Verification items for the finished model (mm, model axes). Coordinates: 2 decimals unless noted, no trailing zeros. Answer in a Markdown table with one row per item.
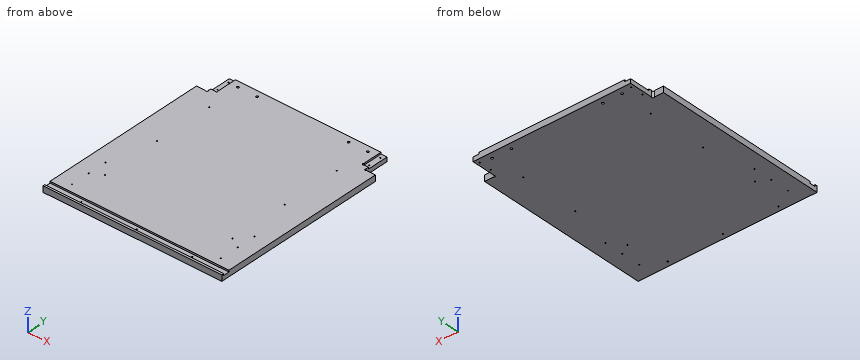
```python
from build123d import *

# Parameters (mm, degrees)
EXTRUDE1_DEPTH     = 17.78
SKETCH4_R          = 3.175
SKETCH4_R_2        = 3.175000003
CUT_EXTRUDE1_DEPTH = 17.78
SKETCH6_R          = 1.5875
CUT_EXTRUDE3_DEPTH = 17.78
SKETCH5_W          = 17.78
SKETCH5_H          = 63.50740041
SKETCH5_H_2        = 63.507400408
CUT_EXTRUDE2_DEPTH = 5.08
SKETCH7_R          = 3.302
CUT_EXTRUDE4_DEPTH = 5.08
SKETCH9_R          = 3.175
CUT_EXTRUDE5_DEPTH = 17.78


with BuildPart() as part:
    # Sketch3 → Extrude1 (new body)
    with BuildSketch(Plane.XY):
        Polygon((10806.641666666, -6342.0625), (11340.041666666, -6342.0625), (11340.041666666, -5818.73683858), (11312.781794728, -5818.73683858), (11308.291666667, -5814.246710519), (11308.291666667, -5742.536838581), (10838.391666667, -5742.536838581), (10838.391666667, -5814.246710519), (10833.901538605, -5818.736838581), (10806.641666666, -5818.736838581), align=None)
    extrude(amount=-EXTRUDE1_DEPTH)

    # Sketch4 → Cut-Extrude1 (cut)
    with BuildSketch(Plane.XY):
        with Locations((11310.536730697, -5816.49177455)):
            Circle(SKETCH4_R)
        with Locations((10836.146602636, -5816.49177455)):
            Circle(SKETCH4_R_2)
    extrude(amount=-CUT_EXTRUDE1_DEPTH, mode=Mode.SUBTRACT)

    # Sketch6 → Cut-Extrude3 (cut)
    with BuildSketch(Plane.XY):
        with Locations((10851.409166666, -6294.4375)):
            Circle(SKETCH6_R)
        with Locations((10908.241666666, -6326.8225)):
            Circle(SKETCH6_R)
        with Locations((11073.341666666, -6326.8225)):
            Circle(SKETCH6_R)
        with Locations((11238.441666666, -6326.8225)):
            Circle(SKETCH6_R)
        with Locations((11295.274166666, -6294.4375)):
            Circle(SKETCH6_R)
        with Locations((11295.274166666, -6237.2875)):
            Circle(SKETCH6_R)
        with Locations((11263.841666666, -6218.2375)):
            Circle(SKETCH6_R)
        with Locations((11295.274166666, -6180.1375)):
            Circle(SKETCH6_R)
        with Locations((11263.841666666, -6040.4375)):
            Circle(SKETCH6_R)
        with Locations((11263.841666666, -5862.6375)):
            Circle(SKETCH6_R)
        with Locations((11299.401666666, -5793.344238991)):
            Circle(SKETCH6_R)
        with Locations((11299.401666666, -5755.236838581)):
            Circle(SKETCH6_R)
        with Locations((10847.281666666, -5755.236838581)):
            Circle(SKETCH6_R)
        with Locations((10847.281666666, -5793.344238991)):
            Circle(SKETCH6_R)
        with Locations((10882.841666666, -6040.4375)):
            Circle(SKETCH6_R)
        with Locations((10851.409166666, -6180.1375)):
            Circle(SKETCH6_R)
        with Locations((10882.841666666, -6218.2375)):
            Circle(SKETCH6_R)
        with Locations((10851.409166666, -6237.2875)):
            Circle(SKETCH6_R)
        with Locations((10882.841666666, -5862.6375)):
            Circle(SKETCH6_R)
    extrude(amount=-CUT_EXTRUDE3_DEPTH, mode=Mode.SUBTRACT)

    # Sketch5 → Cut-Extrude2 (cut)
    with BuildSketch(Plane.XY):
        Polygon((11073.341666666, -6317.9325), (10806.641666666, -6317.9325), (10806.641666666, -6335.7125), (11340.041666666, -6335.7125), (11340.041666666, -6317.9325), align=None)
        with Locations((10847.281666667, -5774.290538786)):
            Rectangle(SKETCH5_W, SKETCH5_H)
        with Locations((11299.401666667, -5774.290538785)):
            Rectangle(SKETCH5_W, SKETCH5_H_2)
    extrude(amount=-CUT_EXTRUDE2_DEPTH, mode=Mode.SUBTRACT)

    # Sketch7 → Cut-Extrude4 (cut)
    with BuildSketch(Plane.XY):
        with Locations((10853.926602637, -5803.79917496)):
            Circle(SKETCH7_R)
        with Locations((11292.756730697, -5803.799174959)):
            Circle(SKETCH7_R)
    extrude(amount=-CUT_EXTRUDE4_DEPTH, mode=Mode.SUBTRACT)

    # Sketch9 → Cut-Extrude5 (cut)
    with BuildSketch(Plane.XY):
        with Locations((10879.616654067, -5760.644320781)):
            Circle(SKETCH9_R)
        with Locations((10936.816666667, -5760.644320781)):
            Circle(SKETCH9_R)
        with Locations((11209.816654067, -5760.644320781)):
            Circle(SKETCH9_R)
        with Locations((11267.016666667, -5760.644320781)):
            Circle(SKETCH9_R)
    extrude(amount=-CUT_EXTRUDE5_DEPTH, mode=Mode.SUBTRACT)


solid = part.part
```
1. Material ranges on probe 1 along X at (y, z) = (-6039, -10.25); probe 2 along Y at (x, z) = (10954.5, -1); probe 3 along X at (y, z) = (-5816, -14.25), recorded low to high. Write a range as from..to.
Findings below:
| item | result |
|---|---|
| probe 1 | x = 10806.64..10882.17, 10883.52..11263.17, 11264.52..11340.04 |
| probe 2 | y = -6342.06..-6335.71, -6317.93..-5742.54 |
| probe 3 | x = 10839.28..11307.4 |
2. Go/stop test with flat-tipped pins: pin 1 (2.5 mm diameter, centred on x = 10847.28, y = -5793.34, fed in from +Z); pin 2 (8.5 mm diameter, centred on x = 11209.82, y = -5760.64, fed in from +Z); pin 3 (9 mm diameter, centred on x = 11328, z = -8.5, fed in from +Y). Record where each tip stops, or that it passes through.
Findings below:
| item | result |
|---|---|
| pin 1 | passes through |
| pin 2 | stops at z = 0 |
| pin 3 | stops at y = -5818.74 |
3. Sectioned sample at A-A, the plane z = -8.75. Count the separate pieces of the cut face and the enclosed holes in it, and give its area (3 significant figures).
Findings below:
| item | result |
|---|---|
| separate pieces | 1 |
| enclosed holes | 23 |
| area | 315,000 mm² |
